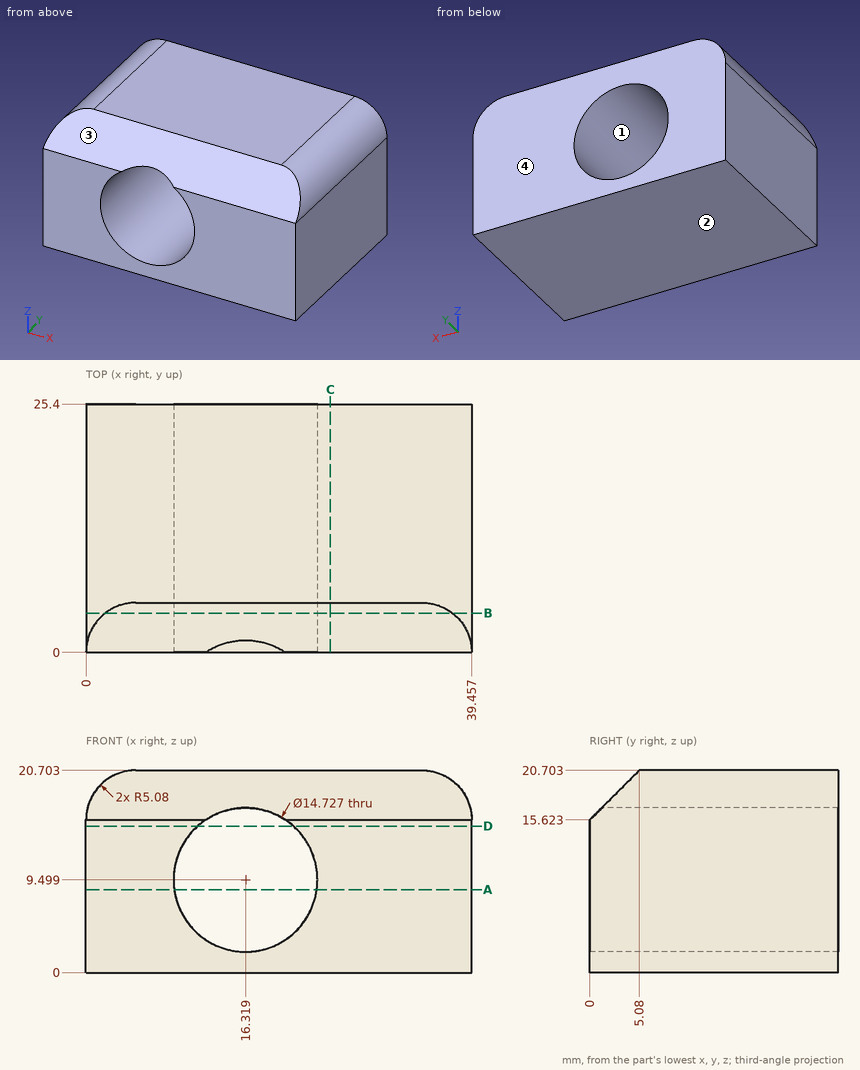
Geometry: see drawing. Coordinates: mm, zero at the bounding-box minimum. Round coordinates to 2 decimals unless told otherwise and drop trailing zeros. Loops run counter-clockwise (first coordinate to the right, second up) from the corner with the lowest first, then second, coordinate; pieces in that order, holes last. Notation, with made-up numbers: M 59,15 L 63,15 A21 cw 63,28 Z; hole C 36,25 d11. An arc over 180 degrees is marked long. Use a Markdown table: item, result. Add a question column.
1. Section query A-A on z = 8.5. Return the cut outline in (x, y).
2. Section query C-C on x = 25. Return the cut outline in (y, z).
3. Section query D-D on z = 15. Return the cut outline in (x, y).
4. Mould query, pull axis Z, two halves, no side actions, for the marked faces 1, 2, 3 and 4. Classes: pulls with the +Z half, pulls with the -Z half, needs draft (parallel to the pull), parting line crosses it, or undercut.
5. Contact query for flat-ended pins moving along their axis: P1, Ø1, axis at x = 27, y = 19.5, coming from the -Z side; P2, Ø2, axis at y = 6, z = 17, coming from the +X side. Output: stop coordinate, or through.
6. Line query: line 1 (Z direction, x = 10.5, y = 7.75) (1 decimal); line 2 (X direction, y = 8.5, z = 6.5) (1 decimal); line 3 (X direction, y = 5, z = 7.25). Output: solid intervals per line, ascending.
7. Section query B-B on y = 4. Return the cut outline in (x, z).
Reported:
| question | item | result |
|---|---|---|
| 1 | outline | M 0,0 L 9.02,0 L 9.02,25.4 L 0,25.4 Z; M 23.61,0 L 39.46,0 L 39.46,25.4 L 23.61,25.4 Z |
| 2 | outline | M 0,0 L 25.4,0 L 25.4,20.7 L 5.08,20.7 L 0,15.62 Z |
| 3 | outline | M 0,0 L 11.42,0 L 11.42,25.4 L 0,25.4 Z; M 21.21,0 L 39.46,0 L 39.46,25.4 L 21.21,25.4 Z |
| 4 | face 1 | undercut |
| 4 | face 2 | pulls with the -Z half |
| 4 | face 3 | pulls with the +Z half |
| 4 | face 4 | needs draft |
| 5 | P1 | stops at z = 0 |
| 5 | P2 | stops at x = 39.44 |
| 6 | line 1 | z = 0 to 5, 14 to 20.7 |
| 6 | line 2 | x = 0 to 9.6, 23 to 39.5 |
| 6 | line 3 | x = 0 to 9.31, 23.33 to 39.46 |
| 7 | outline | M 0,0 L 39.46,0 L 39.46,15.62 A5.08 ccw 37.51,19.62 L 1.95,19.62 A5.08 ccw 0,15.62 Z; hole C 16.32,9.5 d14.73 |
